Input: part model. Units: mm. Frame: model coordinates. A direction names the side the tool comes from. Give positions to 0.01 mm unless a question says otherwise; leave off trailing zeros. Order: outer loops, then holes, each group sorted by start corner. A loop starts at its lowest first (then second) coordinate and runs counter-clockwise, first axis right, second up. Notation, with made-up numbers: (-39.75, -38.5) - (-28.75, -38.5) arc R8 ccw to (-28.75, -32.5) - close; hole circle Ø5 at (-32, 10.25). An arc over 180 degrees is marked (long way). Use a Markdown table: item, result.
from build123d import *

# Parameters (mm, degrees)
F2_R     = 3.5
F3_DEPTH = 25
F4_SIZE  = 2.5
F5_R     = 26
F5_R_2   = 24.5
F6_DEPTH = 1.5
F8_DEPTH = 46.001
F9_DEPTH = 7.8


with BuildPart() as f1:
    # F0 (on Front) → F1 (revolve)
    with BuildSketch(Plane.XZ):
        Polygon((38, 42.8381226957), (22.6, 42.8381226957), (22.6, 39.3381226957), (15.5, 39.3381226957), (15.5, 13.3381226957), (12.7, 13.3381226957), (12.7, -3.1618773043), (18.4, -3.1618773043), (22.3, -3.1618773043), (22.3, 32.8381226957), (38, 32.8381226957), align=None)
    revolve(axis=Axis((0, 0, -18.1553717703), (0, 0, -1)))

    # F2 (on face) → F3 (cut)
    with BuildSketch(Plane.XY.offset(42.8381226957)):
        with Locations((0, 31.75)):
            Circle(F2_R)
        with Locations((0, -31.75)):
            Circle(F2_R)
        with Locations((31.75, 0)):
            Circle(F2_R)
        with Locations((-31.75, 0)):
            Circle(F2_R)
        with Locations((-22.4506403027, 22.4506403027)):
            Circle(F2_R)
        with Locations((22.4506403027, 22.4506403027)):
            Circle(F2_R)
        with Locations((22.4506403027, -22.4506403027)):
            Circle(F2_R)
        with Locations((-22.4506403027, -22.4506403027)):
            Circle(F2_R)
    extrude(amount=-F3_DEPTH, mode=Mode.SUBTRACT)

    # F4
    f4_edges = [f1.edges().sort_by_distance(p)[0] for p in [
        (-22.3, 0, -3.161877),
    ]]
    chamfer(f4_edges, length=F4_SIZE)

    # F5 (on face) → F6 (cut)
    with BuildSketch(Plane(origin=(0, 0, 32.8381226957), x_dir=(1, 0, 0), z_dir=(0, 0, -1))):
        Circle(F5_R)
        Circle(F5_R_2, mode=Mode.SUBTRACT)
    extrude(amount=-F6_DEPTH, mode=Mode.SUBTRACT)

    # F7 (on face) → F8 (cut, through all)
    with BuildSketch(Plane.XY.offset(42.8381226957)):
        Polygon((-17.75567684, 42.8659958362), (-11.2253201513, 27.1003201513), (0, 0), (27.1003201513, 11.2253201513), (39.6317325238, 16.4160011117), (25.7364641875, 40.4654443264), align=None)
    extrude(amount=-F8_DEPTH, mode=Mode.SUBTRACT)

    # F9 (add): a face of the model
    f9_faces = [f1.faces().sort_by_distance(p)[0] for p in [
        (-5.7669841433, -13.9227313326, 13.3381226957),
    ]]
    extrude(f9_faces, amount=F9_DEPTH)


solid = f1.part
1. Section query D-D (z = 3). Return loops of the section in (x, y), then the cut area to 3 significant figures.
Response:
| item | result |
|---|---|
| outline | (-8.53, 20.6) arc R22.3 ccw (long way) to (20.6, 8.53) - (11.73, 4.86) arc R12.7 cw (long way) to (-4.86, 11.73) - close |
| area | 792 mm^2 |
2. Section query C-C (x = 31.75). Return loops of the section in (y, z), then the cut area to 3 significant figures.
Response:
| item | result |
|---|---|
| outline | (-20.88, 32.84) - (-3.5, 32.84) - (-3.5, 42.84) - (-20.88, 42.84) - close; (3.5, 32.84) - (13.15, 32.84) - (13.15, 42.84) - (3.5, 42.84) - close |
| area | 270 mm^2 |
3. Mould query, pull axis Y, two halves, no side actions, for faces 1 (the face through (-5, -26, 32.838)), 2 (the face through (-7.85, -20.873, 16.323)), 3 (the face through (-8.624, -22.932, 33.578)). Classes: pulls with the +Y half, pulls with the -Y half, needs draft (parallel to the pull), parting line crosses it, or undercut.
Response:
| item | result |
|---|---|
| face 1 | needs draft |
| face 2 | parting line crosses it |
| face 3 | undercut |
4. Section query B-B (y = 0). State how many separate pieces and enclosed holes the cut face has, then the cut area to 3 significant figures.
Response:
| item | result |
|---|---|
| separate pieces | 4 |
| enclosed holes | 0 |
| area | 875 mm^2 |
5. Set-up query: faces 4 (the face through (-5.456, -14.508, 30.111)), 5 (the face through (-0.46, -28.28, 37.91)), 6 (the face through (-10, -23, 34.338)). Return all of +Z, -Z, +X, -X, +Y, -Y with unobstructed straight access to the full face (end or side cutting, diameter ignored); none if empty.
Response:
| item | result |
|---|---|
| face 4 | +Z |
| face 5 | +Z, -Z |
| face 6 | -Z |
6. Pin query (flat end, axial travel): pin 1 (21.5 mm diameter, centred on x = -10, y = -6.5, fed in from +Z); pin 2 (10 mm diameter, centred on x = -7.5, z = 37, fed in from -Y); pin 3 (9 mm diameter, centred on x = 0, y = -31.75, fed in from -Z); pin 4 (10 mm diameter, centred on x = -9, y = 14.5, fed in from +Z). Return the tip coordinate at first contact, or that it passes through.
Response:
| item | result |
|---|---|
| pin 1 | stops at z = 42.84 |
| pin 2 | stops at y = -37.92 |
| pin 3 | stops at z = 32.84 |
| pin 4 | stops at z = 39.34 |
7. Section query A-A (x = 0). Return loops of the section in (y, z), then the cut area to 3 significant figures.
Response:
| item | result |
|---|---|
| outline | (-38, 32.84) - (-35.25, 32.84) - (-35.25, 42.84) - (-38, 42.84) - close; (-28.25, 32.84) - (-26, 32.84) - (-26, 34.34) - (-24.5, 34.34) - (-24.5, 32.84) - (-22.3, 32.84) - (-22.3, -0.66) - (-19.8, -3.16) - (-12.7, -3.16) - (-12.7, 21.14) - (-15.5, 21.14) - (-15.5, 39.34) - (-22.6, 39.34) - (-22.6, 42.84) - (-28.25, 42.84) - close |
| area | 438 mm^2 |
8. Material intervals for line 1 along Y through (x, z) = (0, 33.7); line 2 along Y through (x, z) = (0, 39.25); line 3 along X through (y, z) = (-0.5, 35), sorted ascending.
Response:
| item | result |
|---|---|
| line 1 | y = -38 to -35.25, -28.25 to -26, -24.5 to -15.5 |
| line 2 | y = -38 to -35.25, -28.25 to -15.5 |
| line 3 | x = -38 to -35.21, -28.29 to -15.49, 15.49 to 28.29, 35.21 to 38 |
